from build123d import *

# Parameters (mm, degrees)
CROQUIS1_W              = 46.491525
CROQUIS1_H              = 46.794250074
CROQUIS1_W_2            = 44.45
CROQUIS1_H_2            = 42.793750074
SALIENTE_EXTRUIR1_DEPTH = 75.731700962
CROQUIS2_R              = 2.0193
CORTAR_EXTRUIR1_DEPTH   = 92.89220798


with BuildPart() as part:
    # Croquis1 → Saliente-Extruir1 (new body)
    with BuildSketch(Plane.XY):
        Rectangle(CROQUIS1_W, CROQUIS1_H)
        Rectangle(CROQUIS1_W_2, CROQUIS1_H_2, mode=Mode.SUBTRACT)
    extrude(amount=SALIENTE_EXTRUIR1_DEPTH)

    # Croquis2 → Cortar-Extruir1 (cut, through all)
    with BuildSketch(Plane(origin=(-23.2457625, 0, 0), x_dir=(0, 1, 0), z_dir=(-1, 0, 0))):
        with Locations(Location((12.699999873, -65.456700938, 0), (0, 0, 270))):
            Circle(CROQUIS2_R)
        with Locations(Location((-12.699999873, -65.456700938, 0), (0, 0, 270))):
            Circle(CROQUIS2_R)
        with Locations(Location((-12.699999873, -8.306700938, 0), (0, 0, 270))):
            Circle(CROQUIS2_R)
        with Locations(Location((12.699999873, -8.306700938, 0), (0, 0, 270))):
            Circle(CROQUIS2_R)
    extrude(amount=-CORTAR_EXTRUIR1_DEPTH, mode=Mode.SUBTRACT)


solid = part.part
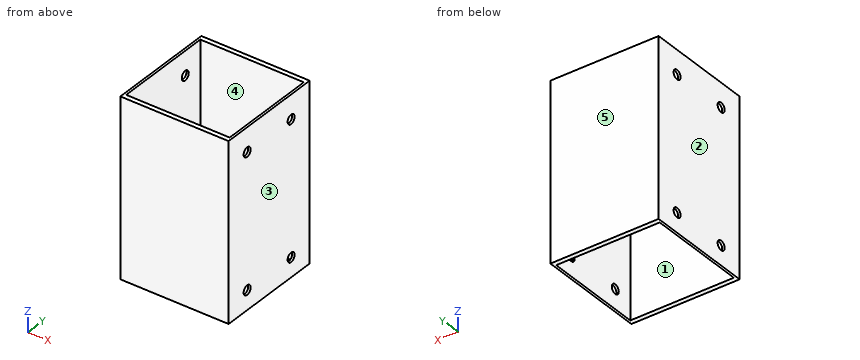
Build history of the part. All positions in model axes, mm. Face numbers are marked on the shaded views. A direction names the side the tool comes from. Coordinates: 2 decimals unless noted, no trailing zeros. Order: outer loops, then holes, each group sorted by start corner. A loop starts at its lowest first (then second) coordinate and runs counter-clockwise, first axis right, second up. Notation, with made-up numbers: (-9, -7.75) - (44, -7.75) arc R25 ccw to (44, 8.25) - close; hole circle Ø6 at (67, 26.5). An arc over 180 degrees is marked (long way). Write item = value, one per line. Start each with the question number.
1) Two-plate mould, pull along Y, no slides. Class the marked faces 3, 4 and 5: pulls with the +Y half, pulls with the -Y half, needs draft (parallel to the pull), parting line crosses it, or undercut.
2) Saw through at D-D on y = 12.7. Write the cut outline in (x, z) (3 decimals).
3) Saw through at A-A on x = -2. Write the cut outline in (y, z).
4) Saw through at C-C on z = 48. Write the cut outline in (x, y) (3 decimals).
5) 3-axis set-ups, long thin cutter, end or side, ignore diameter. For the marked faces 1 and 2: which of +Z, -Z, +X, -X, +Y, -Y reach the whole face in a straight line?
6) Wall check: line 1 along Y through (x, z) = (-13, 46); line 2 along X through (y, z) = (-8, 48.5) (3 decimals). Give the ranges that are in metal, low to high. Write a range as from..to.
7) Saw through at B-B on y = 20.5. Write the cut outline in (x, z) (3 decimals).
From the geometry:
q1.face_3 = needs draft
q1.face_4 = undercut
q1.face_5 = pulls with the +Y half
q2.outline = (-23.246, 0) - (-22.225, 0) - (-22.225, 6.287) - (-23.246, 6.287) - close; (-23.246, 10.326) - (-22.225, 10.326) - (-22.225, 63.437) - (-23.246, 63.437) - close; (-23.246, 67.476) - (-22.225, 67.476) - (-22.225, 75.732) - (-23.246, 75.732) - close; (22.225, 0) - (23.246, 0) - (23.246, 6.287) - (22.225, 6.287) - close; (22.225, 10.326) - (23.246, 10.326) - (23.246, 63.437) - (22.225, 63.437) - close; (22.225, 67.476) - (23.246, 67.476) - (23.246, 75.732) - (22.225, 75.732) - close
q3.outline = (-23.4, 0) - (-21.4, 0) - (-21.4, 75.73) - (-23.4, 75.73) - close; (21.4, 0) - (23.4, 0) - (23.4, 75.73) - (21.4, 75.73) - close
q4.outline = (-23.246, -23.397) - (23.246, -23.397) - (23.246, 23.397) - (-23.246, 23.397) - close; hole (-22.225, -21.397) - (22.225, -21.397) - (22.225, 21.397) - (-22.225, 21.397) - close
q5.face_1 = +Z, -Z
q5.face_2 = +Z, -Z, -X, +Y, -Y
q6.line_1 = -23.4..-21.4, 21.4..23.4
q6.line_2 = -23.246..-22.225, 22.225..23.246
q7.outline = (-23.246, 0) - (-22.225, 0) - (-22.225, 75.732) - (-23.246, 75.732) - close; (22.225, 0) - (23.246, 0) - (23.246, 75.732) - (22.225, 75.732) - close
